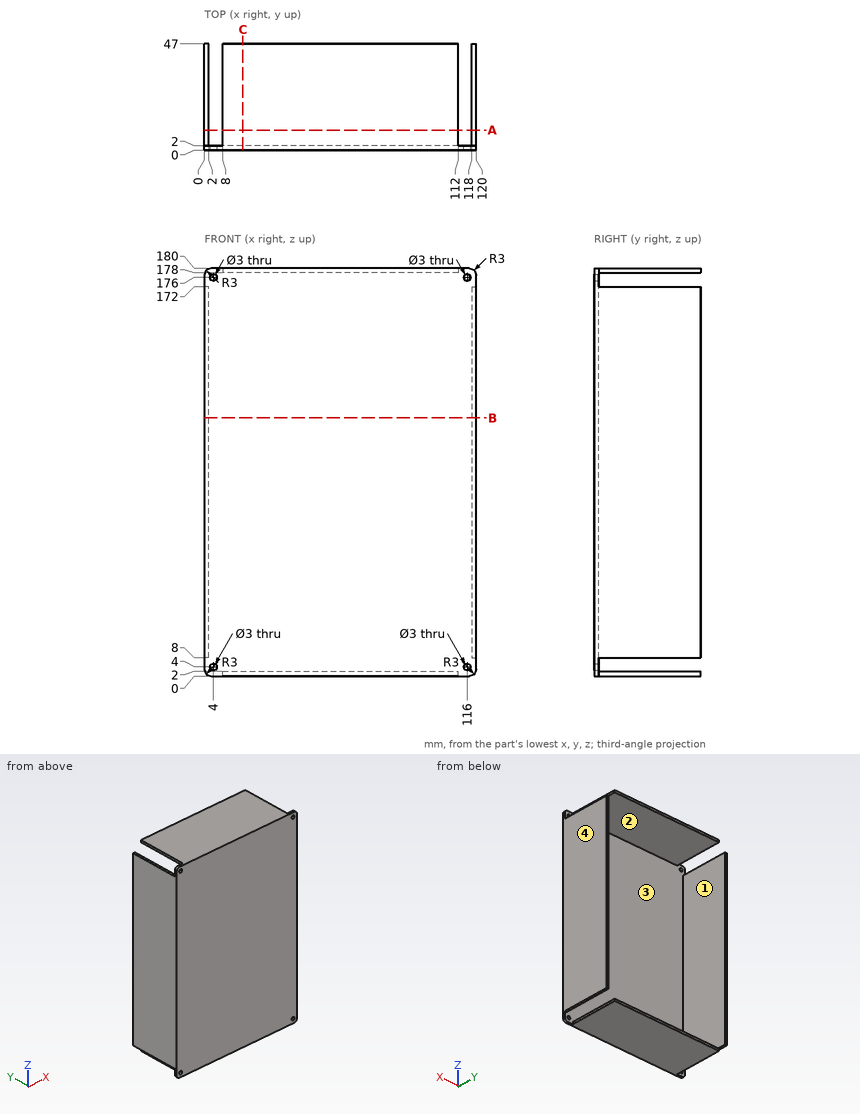
Design review of the part shown in the three views and the two pictorial views. Dimensions are in mm from the part's minimum x, y and z. Give positions to 0.01 mm unless a question says otherwise; leave off trailing zeros. Write each loop counter-clockwise with the first axis right and the second up, starting at its lowest first coordinate (ties: lowest second). Pieces come first, ordered by that corner, then holes. Notation, with made-up numbers: (44.5, 49) - (56.5, 49) arc R24 cw to (56.5, 72) - close; hole circle Ø1 at (86.5, -39). An arc over 180 degrees is marked (long way). Return JSON: item names as keys, results as strings. Group by question number.
(1) To check wall thickness, follow probe 1 along X at (y, z) = (0.9, 176); probe 2 along Z at (x, y) = (4, 1); probe 3 along X at (y, z) = (11, 49.5). State the ranges of each line that lie inside material, in increasing order.
(2) We need section A-A, the plane y = 9. Give the boundary of the cut face in (x, z).
(3) We need section B-B, the plane z = 114. Give the boundary of the cut face in (x, y), then the cut area to 3 significant figures.
(4) Mouldability with a two-part tool opening along X and no side actions: class the marked faces 1, 2, 3 and 4 as +X half, -X half, draft (parallel to the pull), parting line (faces both ways), or undercut.
(5) We need section C-C, the plane x = 17. Give the boundary of the cut face in (y, z), then the cut area to 3 significant figures.
(6) Insertion check: pin 1 (1 mm diameter, centred on y = 24.5, z = 178.5, fed in from -X); pin 2 (1 mm diameter, centred on x = 45, z = 21, fed in from +Y); pin 3 (1 mm diameter, centred on y = 28, z = 179, fed in from +X). Each pin has a flat end and moves straight along its axis. Give the tip position at first contact, or say it passes through.
Reported:
{
 "1": {"probe 1": "x = 0 to 2.5, 5.5 to 114.5, 117.5 to 120", "probe 2": "z = 0 to 2.5, 5.5 to 174.5, 177.5 to 180", "probe 3": "x = 0 to 2, 118 to 120"},
 "2": {"outline": "(0, 8) - (2, 8) - (2, 172) - (0, 172) - close; (8, 0) - (112, 0) - (112, 2) - (8, 2) - close; (8, 178) - (112, 178) - (112, 180) - (8, 180) - close; (118, 8) - (120, 8) - (120, 172) - (118, 172) - close"},
 "3": {"outline": "(0, 0) - (120, 0) - (120, 47) - (118, 47) - (118, 2) - (2, 2) - (2, 47) - (0, 47) - close", "area": "420 mm2"},
 "4": {"face 1": "undercut", "face 2": "draft", "face 3": "undercut", "face 4": "+X half"},
 "5": {"outline": "(0, 0) - (47, 0) - (47, 2) - (2, 2) - (2, 178) - (47, 178) - (47, 180) - (0, 180) - close", "area": "540 mm2"},
 "6": {"pin 1": "stops at x = 8", "pin 2": "stops at y = 2", "pin 3": "stops at x = 112"}
}
